For this review, take the finished solid that the model builds, in its own axes (mm). Face numbers are marked on the shaded views. Round coordinates to 2 decimals unless told otherwise and drop trailing zeros. Order: outer loops, then holes, each group sorted by start corner. A loop starts at its lowest first (then second) coordinate and runs counter-clockwise, first axis right, second up. Notation, with made-up numbers: M -8,21 L 8,21 A33 ccw 8,55 Z; hole C 85.5,11 d7. An arc over 180 degrees is marked long. Answer in a Markdown table with one row per item. Add a question column.
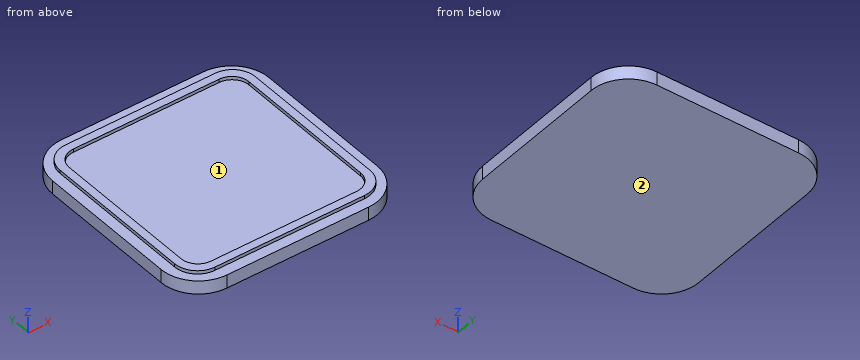
```python
from build123d import *

# Parameters (mm, degrees)
PAD_DEPTH    = 1.6
PAD001_DEPTH = 0.4


with BuildPart() as part:
    # Sketch → Pad (new body)
    with BuildSketch(Plane.XY):
        with BuildLine():
            Line((-8.510103, 12.975), (8.510103, 12.975))
            ThreePointArc((12.975, 8.510103), (11.667262, 11.667262), (8.510103, 12.975))
            Line((12.975, 8.510103), (12.975, -8.510103))
            ThreePointArc((8.510103, -12.975), (11.667262, -11.667262), (12.975, -8.510103))
            Line((8.510103, -12.975), (-8.510103, -12.975))
            ThreePointArc((-12.975, -8.510103), (-11.667262, -11.667262), (-8.510103, -12.975))
            Line((-12.975, -8.510103), (-12.975, 8.510103))
            ThreePointArc((-8.510103, 12.975), (-11.667262, 11.667262), (-12.975, 8.510103))
        make_face()
    extrude(amount=PAD_DEPTH)

    # Sketch001 (on Face10 of Pad) → Pad001 (join)
    with BuildSketch(Plane.XY.offset(1.6)):
        with BuildLine():
            Line((-11.725, 8.992951), (-11.725, -8.99294))
            ThreePointArc((-11.725, -8.99294), (-10.924798, -10.924798), (-8.99294, -11.725))
            Line((-8.99294, -11.725), (8.992951, -11.725))
            ThreePointArc((8.992951, -11.725), (10.924802, -10.924795), (11.725, -8.99294))
            Line((11.725, -8.99294), (11.725, 8.992951))
            ThreePointArc((11.725, 8.992951), (10.924801, 10.924801), (8.992951, 11.725))
            Line((8.992951, 11.725), (-8.99294, 11.725))
            ThreePointArc((-8.99294, 11.725), (-10.924798, 10.924805), (-11.725, 8.992951))
        make_face()
        with BuildLine():
            Line((-8.751524, 10.775), (8.751524, 10.775))
            ThreePointArc((10.775, 8.751524), (10.182338, 10.182338), (8.751524, 10.775))
            Line((10.775, 8.751524), (10.775, -8.751524))
            ThreePointArc((8.751524, -10.775), (10.182338, -10.182338), (10.775, -8.751524))
            Line((8.751524, -10.775), (-8.751524, -10.775))
            ThreePointArc((-10.775, -8.751524), (-10.182338, -10.182338), (-8.751524, -10.775))
            Line((-10.775, -8.751524), (-10.775, 8.751524))
            ThreePointArc((-8.751524, 10.775), (-10.182338, 10.182338), (-10.775, 8.751524))
        make_face(mode=Mode.SUBTRACT)
    extrude(amount=PAD001_DEPTH)


solid = part.part
```
1. The part is to be moulded in two halves that separate along X. For the marked faces 1 and 2, say which applies: pulls with the +X half, pulls with the -X half, needs draft (parallel to the pull), parting line crosses it, or undercut.
2. To check wall thickness, follow probe 1 along X at (y, z) = (5, 1.95) (3 decimals); probe 2 along Z at (x, y) = (5.5, 5). State the ranges of each line that lie inside material, in increasing order. Write a range as [from, to].
3. Clearance check with flat-ended pins moving along their axes: pin 1 Ø12 at (x, y) = (0, -6.5) entering from -Z; pin 2 Ø6.5 at (x, y) = (3, -3.5) entering from +Z. State where each tip first meets the part, or that it passes through.
4. Consider section C-C on z = 0.9. Write out the cut boundary in (x, y) (3 decimals), plus the area to 3 significant figures.
5. Consider section A-A on y = -0.5. Write out the cut boundary in (x, z) (3 decimals).
Solved:
| question | item | result |
|---|---|---|
| 1 | face 1 | undercut |
| 1 | face 2 | needs draft |
| 2 | probe 1 | x = [-11.725, -10.775], [10.775, 11.725] |
| 2 | probe 2 | z = [0, 1.6] |
| 3 | pin 1 | stops at z = 0 |
| 3 | pin 2 | stops at z = 1.6 |
| 4 | outline | M -12.975,-8.51 A4.465 ccw -8.51,-12.975 L 8.51,-12.975 A4.465 ccw 12.975,-8.51 L 12.975,8.51 A4.465 ccw 8.51,12.975 L -8.51,12.975 A4.465 ccw -12.975,8.51 Z |
| 4 | area | 656 mm^2 |
| 5 | outline | M -12.975,0 L 12.975,0 L 12.975,1.6 L 11.725,1.6 L 11.725,2 L 10.775,2 L 10.775,1.6 L -10.775,1.6 L -10.775,2 L -11.725,2 L -11.725,1.6 L -12.975,1.6 Z |
